Build history of the part. All positions in model axes, mm. A direction names the side the tool comes from. Round coordinates to 2 decimals unless told otherwise and drop trailing zeros. Order: outer loops, then holes, each group sorted by start corner. A loop starts at its lowest first (then second) coordinate and runs counter-clockwise, first axis right, second up. Notation, with made-up numbers: M 13,-17.5 L 67,-17.5 A21 cw 67,3.5 Z; hole C 2,36.25 d9. An arc over 180 degrees is marked long. Use CSV: the item, a comma, the result in double quotes.
from build123d import *

# Parameters (mm, degrees)
SKETCH_1_R          = 18.5
EXTRUDE_1_DEPTH     = 22.7
SKETCH_2_R          = 16.5
EXTRUDE_2_DEPTH     = 22.7
SKETCH_3_R          = 6
EXTRUDE_3_DEPTH     = 6
SKETCH_4_R          = 3
EXTRUDE_4_DEPTH     = 15.5
SKETCH_5_W          = 14.350775589
SKETCH_5_H          = 3.642889188
CUT_EXTRUDE_1_DEPTH = 12
SKETCH_6_R          = 1.6
CUT_EXTRUDE_2_DEPTH = 10


with BuildPart() as part:
    # 草图1 → 凸台-拉伸1 (new body)
    with BuildSketch(Plane.XY):
        Circle(SKETCH_1_R)
    extrude(amount=EXTRUDE_1_DEPTH)

    # 草图2 → 凸台-拉伸2 (add)
    with BuildSketch(Plane.XY.offset(22.7)):
        Circle(SKETCH_2_R)
    extrude(amount=EXTRUDE_2_DEPTH)

    # 草图3 → 凸台-拉伸3 (add)
    with BuildSketch(Plane(origin=(0, 0, 0), x_dir=(-1, 0, 0), z_dir=(0, 0, -1))):
        with Locations(Location((0, 7, 0), (0, 0, 180))):
            Circle(SKETCH_3_R)
    extrude(amount=EXTRUDE_3_DEPTH)

    # 草图4 → 凸台-拉伸4 (add)
    with BuildSketch(Plane(origin=(0, 0, -6), x_dir=(-1, 0, 0), z_dir=(0, 0, -1))):
        with Locations((0, 7)):
            Circle(SKETCH_4_R)
    extrude(amount=EXTRUDE_4_DEPTH)

    # 草图5 → 切除-拉伸1 (cut)
    with BuildSketch(Plane(origin=(0, 0, -21.5), x_dir=(-1, 0, 0), z_dir=(0, 0, -1))):
        with Locations((0.938319943, 11.321444594)):
            Rectangle(SKETCH_5_W, SKETCH_5_H)
    extrude(amount=-CUT_EXTRUDE_1_DEPTH, mode=Mode.SUBTRACT)

    # 草图6 → 切除-拉伸2 (cut)
    with BuildSketch(Plane(origin=(0, 0, 0), x_dir=(-1, 0, 0), z_dir=(0, 0, -1))):
        with Locations((0, 15.5)):
            Circle(SKETCH_6_R)
        with Locations((13.423393759, 7.75)):
            Circle(SKETCH_6_R)
        with Locations((13.423393759, -7.75)):
            Circle(SKETCH_6_R)
        with Locations((0, -15.5)):
            Circle(SKETCH_6_R)
        with Locations((-13.423393759, -7.75)):
            Circle(SKETCH_6_R)
        with Locations((-13.423393759, 7.75)):
            Circle(SKETCH_6_R)
    extrude(amount=-CUT_EXTRUDE_2_DEPTH, mode=Mode.SUBTRACT)


solid = part.part
(1) Cut at B-B, the plane x = 13.5. Give the cut face in (y, z), and give its area (3 significant figures).
Answer block:
outline,"M -12.65,0 L -9.35,0 L -9.35,10 L -6.15,10 L -6.15,0 L 6.15,0 L 6.15,10 L 9.35,10 L 9.35,0 L 12.65,0 L 12.65,22.7 L 9.49,22.7 L 9.49,45.4 L -9.49,45.4 L -9.49,22.7 L -12.65,22.7 Z"
area,"941 mm²"
(2) Drop flat-ended pins along their axis: pin 1 (2 mm diameter, centred on x = -4, y = -3, fed in from -Z); pin 2 (1.6 mm diameter, centred on x = -13.5, y = -7.5, fed in from -Z); pin 3 (1.5 mm diameter, centred on x = 4, y = 11.5, fed in from -Z). Give the stop position or say it passes through.
Answer block:
pin 1,"stops at z = 0"
pin 2,"stops at z = 10"
pin 3,"stops at z = -6"
(3) Cut at D-D, the plane y = 7.75. Give the cut face in (x, z), and give its area (3 significant figures).
Answer block:
outline,"M -16.8,0 L -15.02,0 L -15.02,10 L -11.82,10 L -11.82,0 L -5.95,0 L -5.95,-6 L -2.9,-6 L -2.9,-21.5 L 2.9,-21.5 L 2.9,-6 L 5.95,-6 L 5.95,0 L 11.82,0 L 11.82,10 L 15.02,10 L 15.02,0 L 16.8,0 L 16.8,22.7 L 14.57,22.7 L 14.57,45.4 L -14.57,45.4 L -14.57,22.7 L -16.8,22.7 Z"
area,"1,520 mm²"
(4) Cut at A-A, the plane y = 0. Give the cut face in (x, z).
Answer block:
outline,"M -18.5,0 L 18.5,0 L 18.5,22.7 L 16.5,22.7 L 16.5,45.4 L -16.5,45.4 L -16.5,22.7 L -18.5,22.7 Z"
(5) Tool access for faces 5 (the face through (-17, 0, 22.7)), 6 (the face through (0, -15, 10)), 7 (the face through (0, 7, -21.5)): list every direction of +Z, -Z, +X, -X, +Y, -Y with a clear straight run to the whole face (end or side of a thin tool).
Answer block:
face 5,"+Z"
face 6,"-Z"
face 7,"-Z, +X, -X, +Y, -Y"
(6) Wall check: line 1 (Y direction, x = 0, z = 6); line 2 (X direction, y = 7, z = 5); line 3 (Z direction, x = 10.5, y = -0.5). Give the ranges that are in metal, low to high. Write a range as from..to.
Answer block:
line 1,"y = -18.5..-17.1, -13.9..13.9, 17.1..18.5"
line 2,"x = -17.12..-14.84, -12.01..12.01, 14.84..17.12"
line 3,"z = 0..45.4"
(7) Two-plate mould, pull along Y, no slides. Class faces 1 (the face through (-11.825, 7.82, 4.93)), 2 (the face through (0, 9.5, -16)), 3 (the face through (15.24, -6.32, 33.89)), 4 (the face through (13, 8, 10)): released by +Y, released by -Y, zero draft, split by the parting line, or undercut.
Answer block:
face 1,"undercut"
face 2,"released by +Y"
face 3,"split by the parting line"
face 4,"undercut"
(8) Cut at C-C, the plane z = 36. Give the cut face in (x, y), and give its area (3 significant figures).
Answer block:
outline,"C 0,0 d33"
area,"855 mm²"
